Verification items for the finished model (mm, model axes). Give positions to 0.01 mm unless a question says otherwise; leave off trailing zeros. Order: outer loops, then holes, each group sorted by start corner. A loop starts at its lowest first (then second) coordinate and runs counter-clockwise, first axis right, second up. Notation, with made-up numbers: (78, 10) - (94, 10) arc R11 cw to (94, 30) - close; hole circle Ø1 at (14, 14.5). An arc over 180 degrees is marked (long way). Answer as a JSON object with one key per item and string values.
```python
from build123d import *

# Parameters (mm, degrees)
AUFSATZ_LINEAR_AUSTRAGEN1_DEPTH      = 10
AUFSATZ_LINEAR_AUSTRAGEN1_DEPTH_BACK = 10
SKIZZE1_R                            = 8
F_6_0_6_DURCHMESSER_BOHRUNG1_D       = 6
F_6_0_6_DURCHMESSER_BOHRUNG1_DEPTH   = 8.197418143
F_6_0_6_DURCHMESSER_BOHRUNG1_TIP     = 1.802581857
F_5_0_5_DURCHMESSER_BOHRUNG5_D       = 5
F_5_0_5_DURCHMESSER_BOHRUNG5_DEPTH   = 18.497848452
F_5_0_5_DURCHMESSER_BOHRUNG5_TIP     = 1.502151548


with BuildPart() as part:
    # Skizze1 → Aufsatz-Linear austragen1 (new, two sides: drawn at the far end of the back side and taken through both)
    with BuildSketch(Plane.XY.offset(-AUFSATZ_LINEAR_AUSTRAGEN1_DEPTH_BACK)):
        Circle(SKIZZE1_R)
    extrude(amount=AUFSATZ_LINEAR_AUSTRAGEN1_DEPTH + AUFSATZ_LINEAR_AUSTRAGEN1_DEPTH_BACK)

    # Ø6.0 (6) Durchmesser Bohrung1
    with Locations(Plane.XY.offset(10)):
        with Locations((0, 0)):
            Hole(F_6_0_6_DURCHMESSER_BOHRUNG1_D / 2, depth=F_6_0_6_DURCHMESSER_BOHRUNG1_DEPTH)
            with Locations((0, 0, -(F_6_0_6_DURCHMESSER_BOHRUNG1_DEPTH + F_6_0_6_DURCHMESSER_BOHRUNG1_TIP / 2))):  # 118° drill point
                Cone(0, F_6_0_6_DURCHMESSER_BOHRUNG1_D / 2, F_6_0_6_DURCHMESSER_BOHRUNG1_TIP, mode=Mode.SUBTRACT)

    # Ø5.0 (5) Durchmesser Bohrung5
    with Locations(Plane(origin=(0, 0, -10), x_dir=(-1, 0, 0), z_dir=(0, 0, -1))):
        with Locations((0, 0)):
            Hole(F_5_0_5_DURCHMESSER_BOHRUNG5_D / 2, depth=F_5_0_5_DURCHMESSER_BOHRUNG5_DEPTH)
            with Locations((0, 0, -(F_5_0_5_DURCHMESSER_BOHRUNG5_DEPTH + F_5_0_5_DURCHMESSER_BOHRUNG5_TIP / 2))):  # 118° drill point
                Cone(0, F_5_0_5_DURCHMESSER_BOHRUNG5_D / 2, F_5_0_5_DURCHMESSER_BOHRUNG5_TIP, mode=Mode.SUBTRACT)


solid = part.part
```
(1) Release check for a two-part mould opening along X. For faces 1 (the flat face through (3.4, 0.1, 10)), 2 (the cylindrical face through (3, 0, 6)), 3 (the cylindrical face through (-1.73, -7.81, -0.14)) record: pulls with the +X half, pulls with the -X half, needs draft (parallel to the pull), parting line crosses it, or undercut.
Computed values:
{"face 1": "needs draft", "face 2": "undercut", "face 3": "parting line crosses it"}
(2) Section check D-D (y = -6.5). Record the cut outline in (x, z).
Computed values:
{"outline": "(-4.66, -10) - (4.66, -10) - (4.66, 10) - (-4.66, 10) - close"}
(3) Section check A-A (x = 0). Record the cut outline in (y, z).
Computed values:
{"outline": "(-8, -10) - (-2.5, -10) - (-2.5, 1.5) - (-3, 1.8) - (-3, 10) - (-8, 10) - close; (2.5, -10) - (8, -10) - (8, 10) - (3, 10) - (3, 1.8) - (2.5, 1.5) - close"}
(4) Material ranges on line 1 along Y through (x, z) = (0, -6.5); line 2 along Y through (x, z) = (0, 4); line 3 along X through (y, z) = (-1, 2.5), recorded low to high. Write a range as [from, to].
Computed values:
{"line 1": "y = [-8, -2.5], [2.5, 8]", "line 2": "y = [-8, -3], [3, 8]", "line 3": "x = [-7.94, -2.83], [2.83, 7.94]"}
(5) Section check C-C (z = -4). Record the cut outline in (x, y), then the cut area to 3 significant figures.
Computed values:
{"outline": "circle Ø16 at (0, 0); hole circle Ø5 at (0, 0)", "area": "181 mm²"}
(6) Gauge pin test, flat ends, axial feed: pin 1 Ø3 at (x, y) = (0, 0) entering from -Z; pin 2 Ø3 at (y, z) = (-4, -7) entering from -X; pin 3 Ø4 at (x, z) = (4.5, 0.5) entering from -Y; pin 4 Ø5 at (y, z) = (-4.5, 1) entering from +X. Record the tip position at first contact, or that the pin passes through.
Computed values:
{"pin 1": "passes through", "pin 2": "stops at x = -7.6", "pin 3": "stops at y = -7.6", "pin 4": "stops at x = 7.75"}
